Design review of the part built by this model. Coordinates are the model's own, in mm. Coordinates: 2 decimals unless noted, no trailing zeros. Write each loop counter-clockwise with the first axis right and the second up, starting at its lowest first coordinate (ties: lowest second). Pieces come first, ordered by that corner, then holes. Notation, with made-up numbers: M -12,32.5 L 30,32.5 A25 cw 30,61.5 Z; hole C 39.5,-14 d10. An arc over 180 degrees is marked long. Write item = value, one per line.
```python
from build123d import *

# Parameters (mm, degrees)
SKETCH_1_R          = 12.5
SKETCH_1_R_2        = 10.2
EXTRUDE_1_DEPTH     = 30
EXTRUDE_START       = 10
SKETCH_2_R          = 12.5
EXTRUDE_2_DEPTH     = 10
SKETCH_3_R          = 3.1
CUT_EXTRUDE_1_DEPTH = 15
CHAMFER_1_SIZE      = 0.5
CUT_EXTRUDE_START   = -1
SKETCH_4_R          = 10.2
CUT_EXTRUDE_2_DEPTH = 1
SKETCH_5_R          = 1.05
CUT_EXTRUDE_3_DEPTH = 6


with BuildPart() as part:
    # 草图1 → 凸台-拉伸1 (new body)
    with BuildSketch(Plane(origin=(0, 0, 0), x_dir=(0, 0, -1), z_dir=(1, 0, 0))):
        Circle(SKETCH_1_R)
        Circle(SKETCH_1_R_2, mode=Mode.SUBTRACT)
    extrude(amount=EXTRUDE_1_DEPTH)

    # 草图2 → 凸台-拉伸2 (add)
    with BuildSketch(Plane.ZY.offset(EXTRUDE_START)):
        Circle(SKETCH_2_R)
    extrude(amount=-EXTRUDE_2_DEPTH)

    # 草图3 → 切除-拉伸1 (cut, symmetric)
    with BuildSketch(Plane(origin=(0, 0, 0), x_dir=(1, 0, 0), z_dir=(0, 1, 0))):
        with Locations(Location((20, 0, 0), (0, 0, 270))):
            Circle(SKETCH_3_R)
    extrude(amount=CUT_EXTRUDE_1_DEPTH, both=True, mode=Mode.SUBTRACT)

    # 倒角1
    chamfer_1_edges = [part.edges().sort_by_distance(p)[0] for p in [
        (30, 0, 12.5),
    ]]
    chamfer(chamfer_1_edges, length=CHAMFER_1_SIZE)

    # 草图4 → 切除-拉伸2 (cut)
    with BuildSketch(Plane(origin=(0, 0, 0), x_dir=(0, 0, -1), z_dir=(1, 0, 0)).offset(CUT_EXTRUDE_START)):
        Circle(SKETCH_4_R)
    extrude(amount=CUT_EXTRUDE_2_DEPTH, mode=Mode.SUBTRACT)

    # 草图5 → 切除-拉伸3 (cut)
    with BuildSketch(Plane.ZY.offset(10)):
        with Locations((9.53, 0)):
            Circle(SKETCH_5_R)
        with Locations((4.765, -8.253222098)):
            Circle(SKETCH_5_R)
        with Locations((-4.765, -8.253222098)):
            Circle(SKETCH_5_R)
        with Locations((-9.53, 0)):
            Circle(SKETCH_5_R)
        with Locations((-4.765, 8.253222098)):
            Circle(SKETCH_5_R)
        with Locations((4.765, 8.253222098)):
            Circle(SKETCH_5_R)
    extrude(amount=-CUT_EXTRUDE_3_DEPTH, mode=Mode.SUBTRACT)


solid = part.part
```
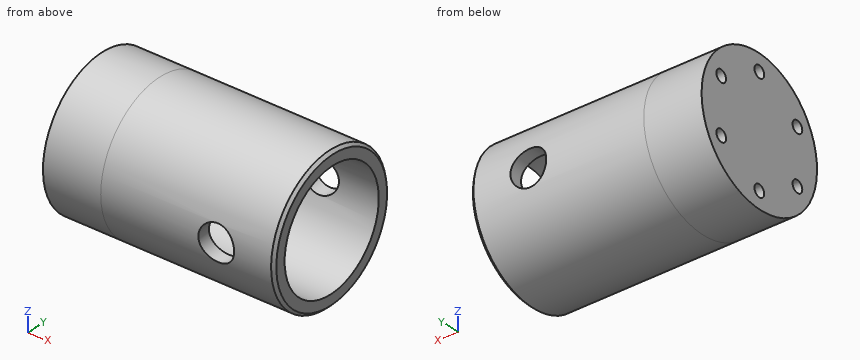
Q1. Consider section C-C, the plane y = 0. State the section outline as (x, z) points.
Check result:
outline = M -10,-12.5 L 29.5,-12.5 L 30,-12 L 30,-10.2 L -1,-10.2 L -1,10.2 L 30,10.2 L 30,12 L 29.5,12.5 L -10,12.5 L -10,10.58 L -4,10.58 L -4,8.48 L -10,8.48 L -10,-8.48 L -4,-8.48 L -4,-10.58 L -10,-10.58 Z
Q2. Wall thickness on line 1 (X direction, y = -11.05, z = 0); line 2 (Y direction, x = -7, z = -5.5); line 3 (Y direction, x = 24, z = -0.25): over which ranges is each line inside the solid? List them lowest first.
Check result:
line_1 = -10 to 16.9, 23.1 to 30
line_2 = -11.22 to -9, -7.5 to 7.5, 9 to 11.22
line_3 = -12.5 to -10.2, 10.2 to 12.5
Q3. Consider section D-D, the plane x = 5. State the section outline as (y, z) points.
Check result:
outline = C 0,0 d25; hole C 0,0 d20.4
Q4. Consider section B-B, the plane x = 20. State the section outline as (y, z) points, and give its area (3 significant figures).
Check result:
outline = M -12.11,-3.1 A12.5 ccw 12.11,-3.1 L 9.72,-3.1 A10.2 cw -9.72,-3.1 Z; M -12.11,3.1 L -9.72,3.1 A10.2 cw 9.72,3.1 L 12.11,3.1 A12.5 ccw Z
area = 135 mm²
Q5. Consider section A-A, the plane z = 0. State the section outline as (x, y) points.
Check result:
outline = M -10,-12.5 L 16.9,-12.5 L 16.9,-10.2 L -1,-10.2 L -1,10.2 L 16.9,10.2 L 16.9,12.5 L -10,12.5 Z; M 23.1,-12.5 L 29.5,-12.5 L 30,-12 L 30,-10.2 L 23.1,-10.2 Z; M 23.1,10.2 L 30,10.2 L 30,12 L 29.5,12.5 L 23.1,12.5 Z
Q6. For P1, Ø1, axis at y = 0.5, z = 9.5, coming from the -X side; P2, Ø1.5, axis at x = -4, z = 1, coming from the -Y side; P3, Ø1, axis at x = 19.5, y = 1.5, coming from the +Z side, all flat-tipped, find the tip position at first contact; note any pin that passes through.
Check result:
P1 = -4
P2 = -12.5
P3 = 12.46
